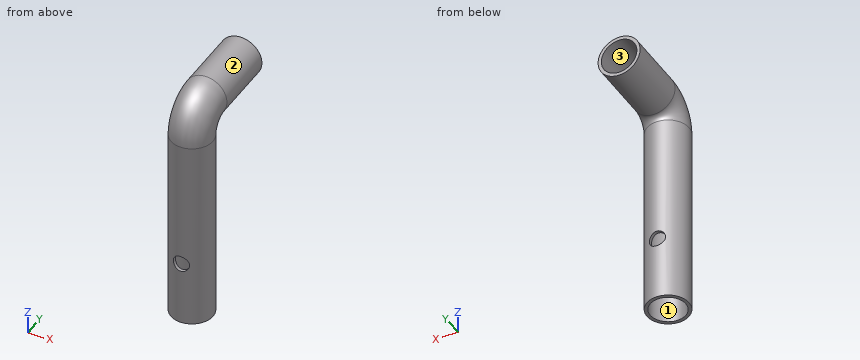
from build123d import *

# Parameters (mm, degrees)
SWEEP5_PROFILE_R        = 6.5
CUT_SWEEP1_PROFILE_R    = 5.5
CUT_EXTRUDE1_DEPTH      = 80.852990027
CUT_EXTRUDE1_DEPTH_BACK = 80.852990027
SKETCH30_R              = 2.5


with BuildPart() as part:
    # Sweep5: sweep along a path in Sketch2
    with BuildLine(Plane(origin=(0, 0, 0), x_dir=(0, 0, -1), z_dir=(1, 0, 0))) as sweep5_path:
        Line((0, 0), (-60, 0))
        ThreePointArc((-60, 0), (-65.656854249, 2.343145751), (-68, 8))
        Line((-68, 8), (-68, 28))
    # Sweep5 profile (on start of the path) → Sweep5 (sweep)
    with BuildSketch(Plane(origin=(0, 0, 0), x_dir=(0, 1, 0), z_dir=(0, 0, 1))):
        Circle(SWEEP5_PROFILE_R)
    sweep(path=sweep5_path.line)

    # Cut-Sweep1: sweep along a path in Sketch2_2
    with BuildLine(Plane(origin=(0, 0, 0), x_dir=(0, 0, -1), z_dir=(1, 0, 0))) as cut_sweep1_path:
        Line((0, 0), (-60, 0))
        ThreePointArc((-60, 0), (-65.656854249, 2.343145751), (-68, 8))
        Line((-68, 8), (-68, 28))
    # Cut-Sweep1 profile (on start of the path) → Cut-Sweep1 (sweep, cut)
    with BuildSketch(Plane(origin=(0, 0, 0), x_dir=(0, 1, 0), z_dir=(0, 0, 1))):
        Circle(CUT_SWEEP1_PROFILE_R)
    sweep(path=cut_sweep1_path.line, mode=Mode.SUBTRACT)

    # Sketch30 → Cut-Extrude1 (cut, two sides: drawn at the far end of the back side and taken through both)
    with BuildSketch(Plane(origin=(0, 0, 0), x_dir=(1, 0, 0), z_dir=(0, 1, 0)).offset(-CUT_EXTRUDE1_DEPTH_BACK)):
        with Locations(Location((0, -20, 0), (0, 0, 90))):
            Circle(SKETCH30_R)
    extrude(amount=CUT_EXTRUDE1_DEPTH + CUT_EXTRUDE1_DEPTH_BACK, mode=Mode.SUBTRACT)


solid = part.part
Build history of the part. All positions in model axes, mm. Face numbers are marked on the shaded views. Coordinates: 2 decimals unless noted, no trailing zeros. Order: outer loops, then holes, each group sorted by start corner. A loop starts at its lowest first (then second) coordinate and runs counter-clockwise, first axis right, second up. Notation, with made-up numbers: (74.25, -4.75) - (91.25, -4.75) arc R8 cw to (91.25, 6.25) - close; hole circle Ø7 at (-3.75, 40.5). An arc over 180 degrees is marked (long way). Write each question's results on one line, items separated by ' | '. Start each with the question number.
Item 1: Band-saw the part on B-B on z = 20. Write the cut outline in (x, y).
Item 2: Flat gauge pins, fed straight in: pin 1 (4 mm diameter, centred on x = -3.5, y = 19, fed in from -Z); pin 2 (3 mm diameter, centred on x = 0, z = 20, fed in from +Y); pin 3 (5 mm diameter, centred on y = 8, z = 60, fed in from +X); pin 4 (5 mm diameter, centred on x = -5, z = 25.5, fed in from +Y). Where does each tip first touch, or does it go through?
Item 3: Band-saw the part on C-C on y = 21. Write the cut outline in (x, z), and give its area (3 significant figures).
Item 4: Mould opens along X. For the marked faces 1, 2 and 3 say: released by +X, released by -X, zero draft, split by the parting line, or undercut.
Item 5: Wall check: probe 1 along X at (y, z) = (0, 36.5); probe 2 along Y at (x, z) = (-3.5, 47). Give the ranges that are in metal, low to high. Write a range as [from, to].
Item 6: Band-saw the part on A-A on x = 0. Write the cut outline in (y, z).
Item 7: Band-saw the part on D-D on z = 47. Write the cut outline in (x, y), and give its area (3 significant figures).
Numbers:
1) outline: (-2.5, -6) - (-2.5, -4.9) arc R5.5 cw to (-2.5, 4.9) - (-2.5, 6) arc R6.5 ccw to start; (2.5, -6) arc R6.5 ccw to (2.5, 6) - (2.5, 4.9) arc R5.5 cw to (2.5, -4.9) - close
2) pin 1: z = 61.68 | pin 2: through | pin 3: x = 3.46 | pin 4: y = 6
3) outline: circle Ø13 at (0, 68); hole circle Ø11 at (0, 68) | area: 37.7 mm^2
4) face 1: undercut | face 2: split by the parting line | face 3: undercut
5) probe 1: [-6.5, -5.5], [5.5, 6.5] | probe 2: [-5.48, -4.24], [4.24, 5.48]
6) outline: (-6.5, 0) - (-5.5, 0) - (-5.5, 17.5) - (-6.5, 17.5) - close; (-6.5, 22.5) - (-5.5, 22.5) - (-5.5, 60) arc R13.5 cw to (8, 73.5) - (28, 73.5) - (28, 74.5) - (8, 74.5) arc R14.5 ccw to (-6.5, 60) - close; (5.5, 0) - (6.5, 0) - (6.5, 17.5) - (5.5, 17.5) - close; (5.5, 22.5) - (6.5, 22.5) - (6.5, 60) arc R1.5 cw to (8, 61.5) - (28, 61.5) - (28, 62.5) - (8, 62.5) arc R2.5 ccw to (5.5, 60) - close
7) outline: circle Ø13 at (0, 0); hole circle Ø11 at (0, 0) | area: 37.7 mm^2
